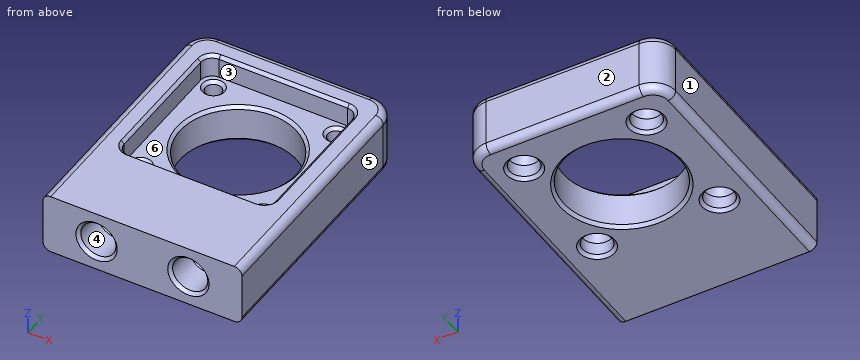
```python
from build123d import *

# Parameters (mm, degrees)
SKETCH1_W           = 26
SKETCH1_H           = 34
BOSS_EXTRUDE1_DEPTH = 8
CUT_EXTRUDE1_REACH  = 24.847
SKETCH2_R           = 7.6
SKETCH2_R_2         = 1.05
SKETCH5_R           = 2.3
CUT_EXTRUDE7_DEPTH  = 4.5
SKETCH6_W           = 19.8
SKETCH6_H           = 19.8
CUT_EXTRUDE8_DEPTH  = 3
SKETCH7_R           = 1.9
CUT_EXTRUDE9_DEPTH  = 3
FILLET1_R           = 3
CHAMFER3_SIZE       = 0.4
FILLET2_R           = 1.5
CHAMFER7_SIZE       = 1
CHAMFER9_SIZE       = 0.4
CHAMFER10_SIZE      = 0.4
FILLET4_R           = 1


with BuildPart() as part:
    # Sketch1 → Boss-Extrude1 (new body)
    with BuildSketch(Plane.XY):
        Rectangle(SKETCH1_W, SKETCH1_H)
    extrude(amount=BOSS_EXTRUDE1_DEPTH)

    # Sketch2 → Cut-Extrude1 (cut, up to next)
    with BuildSketch(Plane.XY.offset(8), mode=Mode.PRIVATE) as cut_extrude1_sk1:
        with Locations((0, 4)):
            Circle(SKETCH2_R)
    cut_extrude1_tool1 = extrude(cut_extrude1_sk1.sketch, amount=-CUT_EXTRUDE1_REACH, mode=Mode.PRIVATE) & part.part
    # Sketch2 → Cut-Extrude1 (cut, up to next)
    with BuildSketch(Plane.XY.offset(8), mode=Mode.PRIVATE) as cut_extrude1_sk2:
        with Locations((-8, 12)):
            Circle(SKETCH2_R_2)
    cut_extrude1_tool2 = extrude(cut_extrude1_sk2.sketch, amount=-CUT_EXTRUDE1_REACH, mode=Mode.PRIVATE) & part.part
    # Sketch2 → Cut-Extrude1 (cut, up to next)
    with BuildSketch(Plane.XY.offset(8), mode=Mode.PRIVATE) as cut_extrude1_sk3:
        with Locations((8, 12)):
            Circle(SKETCH2_R_2)
    cut_extrude1_tool3 = extrude(cut_extrude1_sk3.sketch, amount=-CUT_EXTRUDE1_REACH, mode=Mode.PRIVATE) & part.part
    # Sketch2 → Cut-Extrude1 (cut, up to next)
    with BuildSketch(Plane.XY.offset(8), mode=Mode.PRIVATE) as cut_extrude1_sk4:
        with Locations((8, -4)):
            Circle(SKETCH2_R_2)
    cut_extrude1_tool4 = extrude(cut_extrude1_sk4.sketch, amount=-CUT_EXTRUDE1_REACH, mode=Mode.PRIVATE) & part.part
    # Sketch2 → Cut-Extrude1 (cut, up to next)
    with BuildSketch(Plane.XY.offset(8), mode=Mode.PRIVATE) as cut_extrude1_sk5:
        with Locations((-8, -4)):
            Circle(SKETCH2_R_2)
    cut_extrude1_tool5 = extrude(cut_extrude1_sk5.sketch, amount=-CUT_EXTRUDE1_REACH, mode=Mode.PRIVATE) & part.part
    add(cut_extrude1_tool1.solids().sort_by_distance((0, 4, 8))[0], mode=Mode.SUBTRACT)
    add(cut_extrude1_tool2.solids().sort_by_distance((-8, 12, 8))[0], mode=Mode.SUBTRACT)
    add(cut_extrude1_tool3.solids().sort_by_distance((8, 12, 8))[0], mode=Mode.SUBTRACT)
    add(cut_extrude1_tool4.solids().sort_by_distance((8, -4, 8))[0], mode=Mode.SUBTRACT)
    add(cut_extrude1_tool5.solids().sort_by_distance((-8, -4, 8))[0], mode=Mode.SUBTRACT)

    # Sketch5 → Cut-Extrude7 (cut)
    with BuildSketch(Plane.XZ.offset(17)):
        with Locations(Location((6, 4, 0), (0, 0, 270))):
            Circle(SKETCH5_R)
        with Locations(Location((-6, 4, 0), (0, 0, 90))):
            Circle(SKETCH5_R)
    extrude(amount=-CUT_EXTRUDE7_DEPTH, mode=Mode.SUBTRACT)

    # Sketch6 → Cut-Extrude8 (cut)
    with BuildSketch(Plane.XY.offset(8)):
        with Locations((0, 4)):
            Rectangle(SKETCH6_W, SKETCH6_H)
    extrude(amount=-CUT_EXTRUDE8_DEPTH, mode=Mode.SUBTRACT)

    # Sketch7 → Cut-Extrude9 (cut)
    with BuildSketch(Plane(origin=(0, 0, 0), x_dir=(-1, 0, 0), z_dir=(0, 0, -1))):
        with Locations((-8, 12)):
            Circle(SKETCH7_R)
        with Locations((8, 12)):
            Circle(SKETCH7_R)
        with Locations((-8, -4)):
            Circle(SKETCH7_R)
        with Locations((8, -4)):
            Circle(SKETCH7_R)
    extrude(amount=-CUT_EXTRUDE9_DEPTH, mode=Mode.SUBTRACT)

    # Fillet1
    fillet1_edges = [part.edges().sort_by_distance(p)[0] for p in [
        (-13, 17, 4),
        (13, 17, 4),
    ]]
    fillet(fillet1_edges, radius=FILLET1_R)

    # Chamfer3
    chamfer3_edges = [part.edges().sort_by_distance(p)[0] for p in [
        (6, -12.5, 6.3),
        (6, -17, 6.3),
        (-6, -12.5, 1.7),
        (-6, -17, 1.7),
    ]]
    chamfer(chamfer3_edges, length=CHAMFER3_SIZE)

    # Fillet2
    fillet2_edges = [part.edges().sort_by_distance(p)[0] for p in [
        (9.9, 13.9, 6.5),
        (9.9, -5.9, 6.5),
        (-9.9, -5.9, 6.5),
        (-9.9, 13.9, 6.5),
    ]]
    fillet(fillet2_edges, radius=FILLET2_R)

    # Chamfer7
    # the kernel refuses this chamfer: 1 mm, written as the material it adds along each edge
    with BuildSketch(Plane(origin=(-8, 12, 3), x_dir=(-1, 0, 0), z_dir=(0, -1, 0))) as chamfer7_piece_1_section:
        Polygon((1.9, CHAMFER7_SIZE), (1.9 - CHAMFER7_SIZE, 0), (1.9, 0), align=None)
    chamfer7_piece_1 = revolve(axis=Axis((-8, 12, 3), (0, 0, -1)), mode=Mode.PRIVATE)
    chamfer7_piece_1 = chamfer7_piece_1 - Plane(origin=(-8, 12, 2.4231984), x_dir=(1, 0, 0), z_dir=(0, 0, 1)) * Cylinder(1.05, 8, mode=Mode.PRIVATE)
    add(chamfer7_piece_1)
    with BuildSketch(Plane(origin=(8, 12, 3), x_dir=(-1, 0, 0), z_dir=(0, -1, 0))) as chamfer7_piece_2_section:
        Polygon((1.9, CHAMFER7_SIZE), (1.9 - CHAMFER7_SIZE, 0), (1.9, 0), align=None)
    chamfer7_piece_2 = revolve(axis=Axis((8, 12, 3), (0, 0, -1)), mode=Mode.PRIVATE)
    chamfer7_piece_2 = chamfer7_piece_2 - Plane(origin=(8, 12, 2.4231984), x_dir=(1, 0, 0), z_dir=(0, 0, 1)) * Cylinder(1.05, 8, mode=Mode.PRIVATE)
    add(chamfer7_piece_2)
    with BuildSketch(Plane(origin=(8, -4, 3), x_dir=(-1, 0, 0), z_dir=(0, -1, 0))) as chamfer7_piece_3_section:
        Polygon((1.9, CHAMFER7_SIZE), (1.9 - CHAMFER7_SIZE, 0), (1.9, 0), align=None)
    chamfer7_piece_3 = revolve(axis=Axis((8, -4, 3), (0, 0, -1)), mode=Mode.PRIVATE)
    chamfer7_piece_3 = chamfer7_piece_3 - Plane(origin=(8, -4, 2.4231984), x_dir=(1, 0, 0), z_dir=(0, 0, 1)) * Cylinder(1.05, 8, mode=Mode.PRIVATE)
    add(chamfer7_piece_3)
    with BuildSketch(Plane(origin=(-8, -4, 3), x_dir=(-1, 0, 0), z_dir=(0, -1, 0))) as chamfer7_piece_4_section:
        Polygon((1.9, CHAMFER7_SIZE), (1.9 - CHAMFER7_SIZE, 0), (1.9, 0), align=None)
    chamfer7_piece_4 = revolve(axis=Axis((-8, -4, 3), (0, 0, -1)), mode=Mode.PRIVATE)
    chamfer7_piece_4 = chamfer7_piece_4 - Plane(origin=(-8, -4, 2.4231984), x_dir=(1, 0, 0), z_dir=(0, 0, 1)) * Cylinder(1.05, 8, mode=Mode.PRIVATE)
    add(chamfer7_piece_4)

    # Chamfer9
    chamfer9_edges = [part.edges().sort_by_distance(p)[0] for p in [
        (0, -5.9, 8),
        (-9.9, 4, 8),
        (9.9, 4, 8),
        (0, 13.9, 8),
        (-9.460660172, -5.460660172, 8),
        (9.460660172, -5.460660172, 8),
        (9.460660172, 13.460660172, 8),
        (-9.460660172, 13.460660172, 8),
        (-7.6, 4, 0),
        (-7.6, 4, 5),
        (-6.1, 12, 0),
        (9.9, -4, 0),
        (-6.1, -4, 0),
        (9.9, 12, 0),
    ]]
    chamfer(chamfer9_edges, length=CHAMFER9_SIZE)

    # Chamfer10
    chamfer10_edges = [part.edges().sort_by_distance(p)[0] for p in [
        (-9.05, 12, 5),
        (6.95, 12, 5),
        (6.95, -4, 5),
        (-9.05, -4, 5),
    ]]
    chamfer(chamfer10_edges, length=CHAMFER10_SIZE)

    # Fillet4
    fillet4_edges = [part.edges().sort_by_distance(p)[0] for p in [
        (13, -1.5, 8),
        (13, -1.5, 0),
        (0, 17, 0),
        (0, 17, 8),
        (-13, -1.5, 0),
        (-12.121320344, 16.121320344, 0),
        (12.121320344, 16.121320344, 0),
        (-13, -1.5, 8),
        (-12.121320344, 16.121320344, 8),
        (12.121320344, 16.121320344, 8),
    ]]
    fillet(fillet4_edges, radius=FILLET4_R)


solid = part.part
```
For this review, take the finished solid that the model builds, in its own axes (mm). Face numbers are marked on the shaded views. A direction names the side the tool comes from. Round coordinates to 2 decimals unless told otherwise and drop trailing zeros. Write each loop counter-clockwise with the first axis right and the second up, starting at its lowest first coordinate (ties: lowest second). Pieces come first, ordered by that corner, then holes. Notation, with made-up numbers: (0, -12) -> (20, -12) arc R30 cw to (20, 13) -> close; hole circle Ø9 at (74, 39). An arc over 180 degrees is marked (long way). One line per question, with ' | ' between items. Start each with the question number.
(1) Insertion check: P1, Ø2.5, axis at x = 8, y = 12, coming from the -Z side; P2, Ø3, axis at x = 6.5, z = 3, coming from the -Y side; P3, Ø1, axis at x = -6.5, y = 10.5, coming from the +Z side. Each pin has a flat end and moves straight along its axis. Give the tip position at first contact, or say it passes through.
(2) Add section C-C, the plane y = 4. Write out the cut boundary in (x, z), plus the area to 3 significant figures.
(3) For line 1 along Y through (x, z) = (8, 1); line 2 along X through (y, z) = (-14.4, 4); line 3 along X through (y, z) = (12, 4), list the stretches that pass through material, from the lowest coordinate up. Write a range as from..to.
(4) Mouldability with a two-part tool opening along X and no side actions: class the marked faces 1, 2 and 3 as released by +X, released by -X, zero draft, split by the parting line, or undercut.
(5) Add section B-B, the plane z = 4. Write out the cut boundary in (x, y), plus the area to 3 significant figures.
(6) Tool access review of the marked faces 4, 5 and 6: name each direction out of +Z, -Z, +X, -X, +Y, -Y from which nothing blocks a thin tool from reaching the whole face with its end or side.
(7) Add section A-A, the plane x = 0. Write out the cut boundary in (y, z), plus the area to 3 significant figures.
Answer list:
1) P1: z = 2.65 | P2: y = -16.92 | P3: z = 5
2) outline: (-13, 1) arc R1 ccw to (-12, 0) -> (-8, 0) -> (-7.6, 0.4) -> (-7.6, 4.6) -> (-8, 5) -> (-9.9, 5) -> (-9.9, 7.6) -> (-10.3, 8) -> (-12, 8) arc R1 ccw to (-13, 7) -> close; (7.6, 0.4) -> (8, 0) -> (12, 0) arc R1 ccw to (13, 1) -> (13, 7) arc R1 ccw to (12, 8) -> (10.3, 8) -> (9.9, 7.6) -> (9.9, 5) -> (8, 5) -> (7.6, 4.6) -> close | area: 71.3 mm²
3) line 1: -17..-5.9, -2.1..10.1, 13.9..17 | line 2: -13..-8.3, -3.7..3.7, 8.3..13 | line 3: -13..-9.05, -6.95..6.95, 9.05..13
4) face 1: released by -X | face 2: zero draft | face 3: undercut
5) outline: (-13, -17) -> (-8.7, -17) -> (-8.3, -16.6) -> (-8.3, -12.9) -> (-7.9, -12.5) -> (-4.1, -12.5) -> (-3.7, -12.9) -> (-3.7, -16.6) -> (-3.3, -17) -> (3.3, -17) -> (3.7, -16.6) -> (3.7, -12.9) -> (4.1, -12.5) -> (7.9, -12.5) -> (8.3, -12.9) -> (8.3, -16.6) -> (8.7, -17) -> (13, -17) -> (13, 14) arc R3 ccw to (10, 17) -> (-10, 17) arc R3 ccw to (-13, 14) -> close; hole circle Ø2.1 at (-8, -4); hole circle Ø2.1 at (-8, 12); hole circle Ø15.2 at (0, 4); hole circle Ø2.1 at (8, -4); hole circle Ø2.1 at (8, 12) | area: 643 mm²
6) face 4: -Y | face 5: +Z, -Z, +X, +Y, -Y | face 6: +Z
7) outline: (-17, 0) -> (-4, 0) -> (-3.6, 0.4) -> (-3.6, 4.6) -> (-4, 5) -> (-5.9, 5) -> (-5.9, 7.6) -> (-6.3, 8) -> (-17, 8) -> close; (11.6, 0.4) -> (12, 0) -> (16, 0) arc R1 ccw to (17, 1) -> (17, 7) arc R1 ccw to (16, 8) -> (14.3, 8) -> (13.9, 7.6) -> (13.9, 5) -> (12, 5) -> (11.6, 4.6) -> close | area: 136 mm²
